Verification items for this drawing (mm, ordinates from the low corner). A direction names the side the tool comes from. Coordinates: 2 decimals unless noted, no trailing zeros. Order: outer loops, then holes, each group sorted by start corner. A loop starts at its lowest first (then second) coordinate and runs counter-clockwise, first axis right, second up. Notation, with made-up numbers: (60, -26.75) -> (66, -26.75) arc R30 ccw to (66, -0.75) -> close; hole circle Ø11 at (81.25, 57.5). An arc over 180 degrees is marked (long way). Write item = value, one per line. Start each with the question number.
1. Cross-section at A-A on z = 11. Record the cut outline in (x, y).
2. Thickness scan on line 1 along Y through (x, z) = (10.5, 7.75); line 2 along Y through (x, z) = (27, 11.75); line 3 along X through (y, z) = (20.5, 13.5). Record the ranges inside material, lowest first. Write a range as from..to.
3. Cross-section at B-B on x = 74. Record the cut outline in (y, z).
4. Go/stop test with flat-tipped pins: P1, Ø3, axis at x = 66.5, z = 3.5, coming from the +Y side; P2, Ø1.5, axis at y = 71.5, z = 3.5, coming from the -X side; P3, Ø3, axis at x = 14.5, z = 10, coming from the +Y side; P4, Ø1.5, axis at y = 12, z = 12.5, coming from the -X side. Record where each tip stops, or that it passes through.
5. Set-up check for the marked faces 1 and 2: record each of +Z, -Z, +X, -X, +Y, -Y from which the full face is reachable in a straight line by a thin tool's end or side.
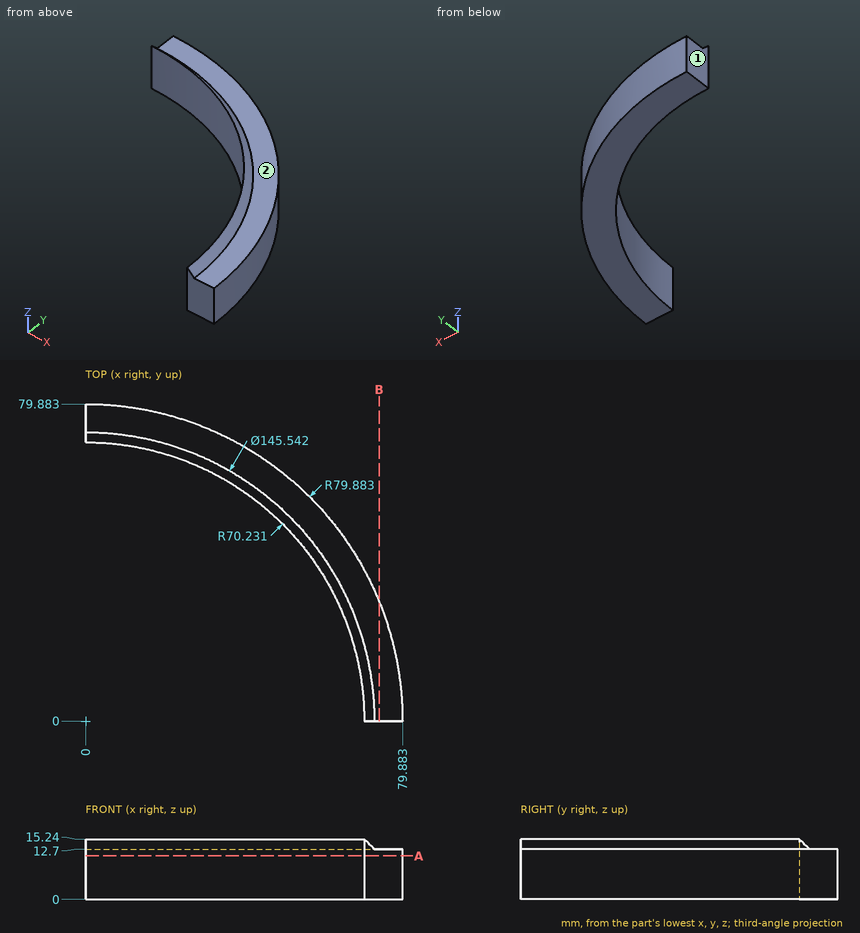
Worked out:
q1.outline = (0, 70.23) arc R70.23 cw to (70.23, 0) -> (79.88, 0) arc R79.88 ccw to (0, 79.88) -> close
q2.line_1 = 69.44..79.19
q2.line_2 = 64.83..75.18
q2.line_3 = 67.17..68.99
q3.outline = (0, 0) -> (30.09, 0) -> (30.09, 12.7) -> (0, 12.7) -> close
q4.P1 = 46.44
q4.P2 = 0
q4.P3 = 78.82
q4.P4 = 69.06
q5.face_1 = +Z, -Z, -X, +Y, -Y
q5.face_2 = +Z, +X, +Y
